Work out the finished part from the listing and answer in its coordinate system (mm). A direction names the side the tool comes from. Round coordinates to 2 decimals unless told otherwise and drop trailing zeros. Order: outer loops, then holes, each group sorted by start corner. A loop starts at its lowest first (then second) coordinate and runs counter-clockwise, first axis right, second up. Notation, with made-up numbers: (-10, 55) - (10, 55) arc R21 ccw to (10, 92) - close; hole circle Ø9 at (82.25, 23). An arc over 180 degrees is marked (long way). Put each result on its own line as item: value.
```python
from build123d import *

# Parameters (mm, degrees)
F0_R     = 29.5141239903
F1_DEPTH = 125
F2_R     = 5
F3_W     = 373.883869499
F3_H     = 179.5099824667
F4_DEPTH = 29.5151239903
F5_T     = -2.5


with BuildPart() as f1:
    # F0 (on Right) → F1 (new body)
    with BuildSketch(Plane.YZ):
        Circle(F0_R)
    extrude(amount=F1_DEPTH)

    # F2
    f2_edges = [f1.edges().sort_by_distance(p)[0] for p in [
        (0, -29.514124, 0),
        (125, -29.514124, 0),
    ]]
    fillet(f2_edges, radius=F2_R)

    # F3 (on Top) → F4 (cut, through all)
    with BuildSketch(Plane.XY):
        with Locations((-27.8811287135, 41.5856614709)):
            Rectangle(F3_W, F3_H)
    extrude(amount=F4_DEPTH, mode=Mode.SUBTRACT)

    # F5
    f5_openings = [f1.faces().sort_by_distance(p)[0] for p in [
        (62.5, 0, 0),
    ]]
    offset(amount=F5_T, openings=f5_openings)


solid = f1.part
```
1) For faces 1 (the flat face through (122.5, 0, -9)), 2 (the flat face through (44, -28, 0)), determine the directions among +Z, -Z, +X, -X, +Y, -Y from which every point of the face is accessible in a straight line to the end or side of a thin tool.
Findings below:
face 1: +Z
face 2: +Z, +X, -X, +Y, -Y
2) Straight lines are drawn through the part: L1, parallel to X at y = 1, z = -14.25; L2, parallel to Z at x = 26, y = -0.5; L3, parallel to Y at x = 113, z = -1.25. For each, find the intervals that lie inside material, in ascending order. Write a range as from..to.
Findings below:
L1: x = 0..2.5, 122.5..125
L2: z = -29.51..-27.01
L3: y = -29.49..-26.99, 26.99..29.49
3) Given pin 1 Ø3 at (x, y) = (72.5, 9.5) entering from +Z; pin 2 Ø2 at (x, z) = (95.5, -22) entering from +Y; pin 3 Ø6 at (x, z) = (32.5, -13.5) entering from -Y, each flat-ended and moving along its own axis, determine where each tip first touches the part or whether it passes through.
Findings below:
pin 1: stops at z = -24.67
pin 2: stops at y = 20.74
pin 3: stops at y = -27.58
4) A cutting plane is placed at B-B on x = 68. Write down the section's boundary in (y, z).
Findings below:
outline: (-29.51, 0) arc R29.51 ccw to (29.51, 0) - (27.01, 0) arc R27.01 cw to (-27.01, 0) - close
5) For a pull along Y with two mould halves and no side action, classify faces 3 (the flat face through (2.5, 0, -9)), 4 (the cylindrical face through (61.695, -0.649, -29.507)), 5 (the flat face through (0, 0, -9)) as pulls with the +Y half, pulls with the -Y half, needs draft (parallel to the pull), parting line crosses it, or undercut.
Findings below:
face 3: undercut
face 4: parting line crosses it
face 5: needs draft
6) A cutting plane is placed at A-A on y = 0. Write down the section's boundary in (x, z).
Findings below:
outline: (0, -24.51) arc R5 ccw to (5, -29.51) - (120, -29.51) arc R5 ccw to (125, -24.51) - (125, 0) - (122.5, 0) - (122.5, -24.51) arc R2.5 cw to (120, -27.01) - (5, -27.01) arc R2.5 cw to (2.5, -24.51) - (2.5, 0) - (0, 0) - close
